Part model, mm, in its own coordinate system. Round coordinates to 2 decimals unless told otherwise and drop trailing zeros. Loops run counter-clockwise (first coordinate to the right, second up) from the corner with the lowest first, then second, coordinate; pieces in that order, holes last.
(1) Cut at C-C on x = 30.5. List the corners of the cut face in (y, z).
(2) Cut at A-A on z = 1.4. List the corners of the cut face in (x, y).
(3) Flat gauge pins, fed straight in: pin 1 (5 mm diameter, centred on x = 58.5, y = 12.5, fed in from +Z); pin 2 (0.5 mm diameter, centred on x = -4.5, z = 1.5, fed in from +Y). Where does each tip first touch, or does it go through?
(4) Probe probe 1 along Z at (x, y) = (61.5, 15); probe 2 along X at (y, z) = (28, 1.2). List the from-to ranges inside material, lowest first.
(5) Cut at B-B on y = 22.5. List the corners of the cut face in (x, z).
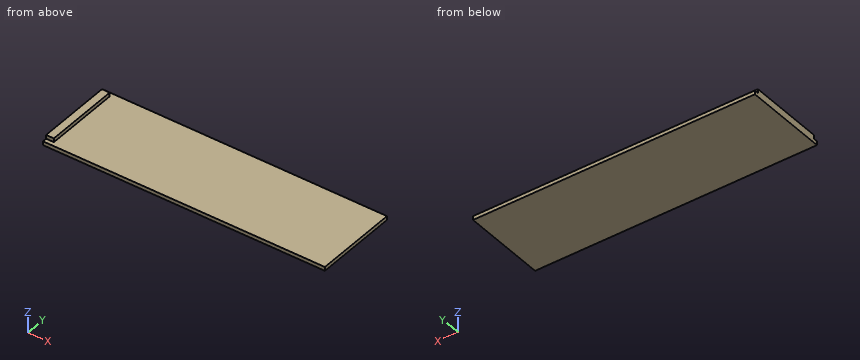
Autodesk Fusion 360 part; units mm, degrees
sketch "Esquisse1" plane through (0, 0, 0) normal (0, 0, 1) x (1, 0, 0)
  line L0 (-5.6946, 30) -> (67.3054, 30)
  line L1 (67.3054, 30) -> (67.3054, 8.2)
  line L2 (67.3054, 8.2) -> (-5.6946, 8.2)
  line L3 (-5.6946, 8.2) -> (-5.6946, 30)
  dimension "d1" = 73
  dimension "d2" = 21.8
extrude "Extrusion1" add sketch "Esquisse1" along normal blind 1
sketch "Esquisse2" plane through (0, 0, 1) normal (0, 0, 1) x (-1, 0, 0)
  line L0 (5.6946, -8.2) -> (-67.3054, -8.2)
  line L1 (-67.3054, -8.2) -> (-67.3054, -30)
  line L2 (-67.3054, -30) -> (5.6946, -30)
  line L3 (5.6946, -30) -> (5.6946, -8.2)
  line L4 (5.6946, -9.3) -> (3.6946, -9.3)
  line L5 (3.6946, -9.3) -> (3.6946, -28.9)
  line L6 (3.6946, -28.9) -> (5.6946, -28.9)
  line L7 (5.6946, -28.9) -> (5.6946, -9.3)
  line L8 (-67.3054, -19.1) -> (5.6946, -19.1) construction
  dimension "d5" = 19.6
  dimension "d8" = 2
extrude "Extrusion2" add sketch "Esquisse2" along normal blind 1 contours L3 L4 L5 L6 L7
equation "d8 = DesignConfigurationRule.64bc9023-8e4e-4cc4-8a85-19370bf7f1c2.dsgcfgrule"
Final values:
1. outline: (8.2, 0) - (30, 0) - (30, 1) - (8.2, 1) - close
2. outline: (-5.69, 9.3) - (-3.69, 9.3) - (-3.69, 28.9) - (-5.69, 28.9) - close
3. pin 1: stops at z = 1
3. pin 2: stops at y = 28.9
4. probe 1: z = 0 to 1
4. probe 2: x = -5.69 to -3.69
5. outline: (-5.69, 0) - (67.31, 0) - (67.31, 1) - (-3.69, 1) - (-3.69, 2) - (-5.69, 2) - close
